from build123d import *

# Parameters (mm, degrees)
SKETCH1_R           = 12.7
BOSS_EXTRUDE1_DEPTH = 139.7
FILLET1_R           = 0.635


with BuildPart() as part:
    # Sketch1 → Boss-Extrude1 (new body)
    with BuildSketch(Plane(origin=(0, 0, 0), x_dir=(1, 0, 0), z_dir=(0, 1, 0))):
        with Locations(Location((0, 0, 0), (0, 0, 270))):
            Circle(SKETCH1_R)
        Polygon((7.478995387, 0), (3.739497694, 6.477), (-3.739497694, 6.477), (-7.478995387, 0), (-3.739497694, -6.477), (3.739497694, -6.477), align=None, mode=Mode.SUBTRACT)
    extrude(amount=BOSS_EXTRUDE1_DEPTH)

    # Fillet1
    fillet1_edges = [part.edges().sort_by_distance(p)[0] for p in [
        (0, 0, -6.477),
        (-5.60924654, 0, -3.2385),
        (-5.60924654, 0, 3.2385),
        (0, 0, 6.477),
        (5.60924654, 139.7, 3.2385),
        (5.60924654, 139.7, -3.2385),
        (0, 139.7, -6.477),
        (-5.60924654, 139.7, -3.2385),
        (-5.60924654, 139.7, 3.2385),
        (0, 139.7, 6.477),
        (0, 0, -12.7),
        (0, 139.7, -12.7),
        (5.60924654, 0, 3.2385),
        (5.60924654, 0, -3.2385),
    ]]
    fillet(fillet1_edges, radius=FILLET1_R)


solid = part.part
The listing builds one solid part. Answer for the finished solid, in the listing's coordinates (mm). A direction names the side the tool comes from. Give positions to 0.01 mm unless a question says otherwise; leave off trailing zeros. Write each loop counter-clockwise with the first axis right and the second up, starting at its lowest first coordinate (ties: lowest second). Pieces come first, ordered by that corner, then holes.
Item 1: Section B-B, the plane y = 72 is taken. Write down the section's boundary in (x, z).
Item 2: Which of the six approach directions +Z, -Z, +X, -X, +Y, -Y give full straight-line access (tool end or side, diameter ignored) to faces 1 (the cylindrical face through (5.795, 139.509, 3.279)), 2 (the cylindrical face through (-5.795, 0.191, -3.279)), 3 (the flat face through (0, 69, 6.477)), 4 (the flat face through (6, 139.7, 5))?
Item 3: Determine the mould class of faces 5 (the flat face through (5.635, 68.881, -3.193)), 6 (the flat face through (6, 0, 5)), 7 (the cylindrical face through (-7.7, 68.9, -10.1)) for opening direction X: released by +X, released by -X, zero draft, split by the parting line, or undercut.
Item 4: Section A-A, the plane x = 0 is taken. Write down the section's boundary in (y, z) (3 decimals), plus the area to 3 significant figures.
Item 5: Find the intervals of material crossed by line 1 along Z through (x, y) = (-0.75, 81); line 2 along X through (y, z) = (15, 3.5); line 3 along X through (y, z) = (58.5, -5), in increasing order.
Item 6: Flat-ended cylindrical pins translate along their axes: P1, Ø3, axis at x = -8, y = 115.5, coming from the +Z side; P2, Ø1, axis at y = 98, z = -10, coming from the +X side; P3, Ø5, axis at x = 6.5, y = 32.5, coming from the -Z side. Find the tip coordinate at first contact, or state that the pin passes through.
Completed:
1. outline: circle Ø25.4 at (0, 0); hole (-7.48, 0) - (-3.74, -6.48) - (3.74, -6.48) - (7.48, 0) - (3.74, 6.48) - (-3.74, 6.48) - close
2. face 1: +Y
2. face 2: -Y
2. face 3: +Y, -Y
2. face 4: +Z, -Z, +X, -X, +Y
3. face 5: undercut
3. face 6: zero draft
3. face 7: split by the parting line
4. outline: (0, -12.065) arc R0.635 ccw to (0.635, -12.7) - (139.065, -12.7) arc R0.635 ccw to (139.7, -12.065) - (139.7, -7.112) arc R0.635 ccw to (139.065, -6.477) - (0.635, -6.477) arc R0.635 ccw to (0, -7.112) - close; (0, 7.112) arc R0.635 ccw to (0.635, 6.477) - (139.065, 6.477) arc R0.635 ccw to (139.7, 7.112) - (139.7, 12.065) arc R0.635 ccw to (139.065, 12.7) - (0.635, 12.7) arc R0.635 ccw to (0, 12.065) - close
4. area: 1,740 mm2
5. line 1: z = -12.68 to -6.48, 6.48 to 12.68
5. line 2: x = -12.21 to -5.46, 5.46 to 12.21
5. line 3: x = -11.67 to -4.59, 4.59 to 11.67
6. P1: stops at z = 10.91
6. P2: stops at x = 8.43
6. P3: stops at z = -12.05
